Autodesk Inventor part; units mm, degrees
ref_plane "YZ Plane" through (0, 0, 0) normal (1, 0, 0) x (0, 1, 0)
ref_plane "XZ Plane" through (0, 0, 0) normal (0, 1, 0) x (-1, 0, 0)
ref_plane "XY Plane" through (0, 0, 0) normal (0, 0, 1) x (1, 0, 0)
sketch "Sketch1" plane through (0, 0, 0) normal (0, 1, 0) x (-1, 0, 0)
  line L0 (0, 0) -> (0, -10) construction
  line L1 (0, -10) -> (2.5, -10)
  line L2 (2.5, -10) -> (2.5, -15)
  line L3 (2.5, -15) -> (5, -15)
  line L4 (5, -15) -> (5, -2)
  line L5 (5, 0) -> (0, 0) construction
  line L6 (0, -10) -> (-2.5, -10)
  line L7 (-2.5, -10) -> (-2.5, -15)
  line L8 (-2.5, -15) -> (-5, -15)
  line L9 (-5, -15) -> (-5, -2)
  line L10 (-5, 0) -> (0, 0) construction
  line L11 (5, 0) -> (5, -2) construction
  line L12 (5, -2) -> (-5, -2)
  dimension "d1" = 10
  dimension "d2" = 2.5
  dimension "d3" = 5
  dimension "d4" = 2.5
  dimension "d7" = 2
revolve "Revolution1" add sketch "Sketch1" angle 360 about axis through (-5, 0, 0) along (1, 0, 0)
fillet "Fillet1" radius 2 2 edges at (-2.5, 0, 10) (2.5, 0, 10)
properties part number "Align_Roller"
Design review of the part built by this model. Coordinates are the model's own, in mm. A direction names the side the tool comes from. Coordinates: 2 decimals unless noted, no trailing zeros. Order: outer loops, then holes, each group sorted by start corner. A loop starts at its lowest first (then second) coordinate and runs counter-clockwise, first axis right, second up. Notation, with made-up numbers: M 4,-4.5 L 37,-4.5 A24 ccw 37,13.5 Z; hole C 10.25,30 d11. An arc over 180 degrees is marked long. Answer as a JSON object with one key per item and string values. Group by question number.
1) For pin 1 (3 mm diameter, centred on x = -2, z = -9.5, fed in from +Y); pin 2 (1 mm diameter, centred on x = -2.5, y = 8, fed in from +Z); pin 3 (2 mm diameter, centred on x = -2.5, z = 2, fed in from -Y), all flat-tipped, find the tip position at first contact; note any pin that passes through.
2) Tool access review of faces 1 (the flat face through (-2.5, 10, 7)), 2 (the cylindrical face through (3.768, 0.66, 14.985)): name each direction out of +Z, -Z, +X, -X, +Y, -Y from which nothing blocks a thin tool from reaching the whole face with its end or side.
3) Add section D-D, the plane y = 12.5. Write out the cut boundary in (x, z), then the cut area to 3 significant figures.
4) Wall thickness on L1, parallel to X at y = -1.75, z = -12; L2, parallel to Y at x = 1.25, z = 0; L3, parallel to Y at x = -2.25, z = 0: over which ranges is each line inside the solid? List them lowest first.
5) Add section A-A, the plane z = 0. Write out the cut boundary in (x, y), then the cut area to 3 significant figures.
6) Mouldability with a two-part tool opening along Z and no side actions: class faces 3 (the cylindrical face through (0, -2, 0)), 4 (the flat face through (2.5, 10, 7)), 5 (the cylindrical face through (0.01, -9.76, 2.17)) as pulls with the +Z half, pulls with the -Z half, needs draft (parallel to the pull), parting line crosses it, or undercut.
7) Add section C-C, the plane x = 4. Write out the cut boundary in (y, z), then the cut area to 3 significant figures.
Computed values:
{
 "1": {"pin 1": "stops at y = 12.63", "pin 2": "stops at z = 12.99", "pin 3": "stops at y = -14.97"},
 "2": {"face 1": "none", "face 2": "+X, -X"},
 "3": {"outline": "M -5,-8.29 L -2.5,-8.29 L -2.5,8.29 L -5,8.29 Z; M 2.5,-8.29 L 5,-8.29 L 5,8.29 L 2.5,8.29 Z", "area": "82.9 mm^2"},
 "4": {"L1": "x = -5 to -2.5, 2.5 to 5", "L2": "y = -10.15 to -2, 2 to 10.15", "L3": "y = -11.03 to -2, 2 to 11.03"},
 "5": {"outline": "M -5,-15 L -2.5,-15 L -2.5,-12 A2 cw -0.5,-10 L 0.5,-10 A2 cw 2.5,-12 L 2.5,-15 L 5,-15 L 5,-2 L -5,-2 Z; M -5,2 L 5,2 L 5,15 L 2.5,15 L 2.5,12 A2 cw 0.5,10 L -0.5,10 A2 cw -2.5,12 L -2.5,15 L -5,15 Z", "area": "213 mm^2"},
 "6": {"face 3": "undercut", "face 4": "needs draft", "face 5": "parting line crosses it"},
 "7": {"outline": "C 0,0 d30; hole C 0,0 d4", "area": "694 mm^2"}
}
